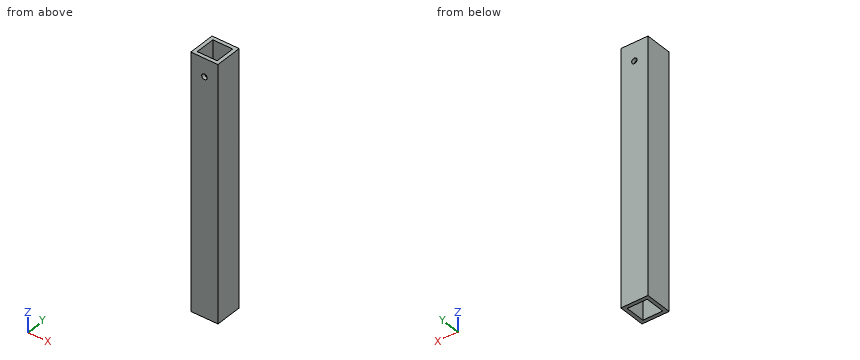
Autodesk Inventor part; units mm, degrees
ref_plane "YZ Plane" through (0, 0, 0) normal (1, 0, 0) x (0, 1, 0)
ref_plane "XZ Plane" through (0, 0, 0) normal (0, 1, 0) x (-1, 0, 0)
ref_plane "XY Plane" through (0, 0, 0) normal (0, 0, 1) x (1, 0, 0)
sketch "Sketch1" plane through (0, 0, 0) normal (0, 0, 1) x (1, 0, 0)
  line L0 (0, 0) -> (15, 0)
  line L1 (15, 0) -> (15, 15)
  line L2 (15, 15) -> (0, 15)
  line L3 (0, 15) -> (0, 0)
  dimension "d0" = 15
  dimension "d1" = 15
extrude "Extrusion1" add sketch "Sketch1" against normal blind 140
shell "Shell1" thickness 2 removed faces 2 at (10, 5, 0) at (10, 5, -140)
sketch "Sketch2" plane through (0, 15, 0) normal (0, 1, 0) x (1, 0, 0)
  line L0 (2, 0) -> (13, 0)
  line L1 (7.5, 0) -> (7.5, 10)
  circle A0 centre (7.5, 10) radius 1.5
  point P0 (0, 0)
  dimension "d5" = 10
  dimension "d6" = 3
extrude "Extrusion2" cut sketch "Sketch2" against normal through all
properties part number "Alumunium Square Tube 14cm"
Could you check a few things on this model? Use its own coordinates, in mm. Give positions to 0.01 mm unless a question says otherwise; leave off trailing zeros. Write each loop counter-clockwise with the first axis right and the second up, starting at its lowest first coordinate (ties: lowest second). Pieces come first, ordered by that corner, then holes. Notation, with made-up numbers: (24, -30) -> (40, -30) arc R31 cw to (40, -2) -> close; hole circle Ø6 at (64, -38.5). An arc over 180 degrees is marked (long way). Answer as a JSON object with one key per item and string values.
Q1. Suppose I cut it at C-C on z = -10. Write out the boundary of the cut face in (x, y).
Taken from the geometry:
{"outline": "(0, 0) -> (6, 0) -> (6, 2) -> (2, 2) -> (2, 13) -> (6, 13) -> (6, 15) -> (0, 15) -> close; (9, 0) -> (15, 0) -> (15, 15) -> (9, 15) -> (9, 13) -> (13, 13) -> (13, 2) -> (9, 2) -> close"}
Q2. Suppose I cut it at D-D on z = -130. Write out the boundary of the cut face in (x, y).
Taken from the geometry:
{"outline": "(0, 0) -> (15, 0) -> (15, 15) -> (0, 15) -> close; hole (2, 2) -> (13, 2) -> (13, 13) -> (2, 13) -> close"}
Q3. Please list where these lines run through material, in increasing order: L1, parallel to Y at x = 5, z = -30; L2, parallel to Z at x = 7.5, y = 1.35.
Taken from the geometry:
{"L1": "y = 0 to 2, 13 to 15", "L2": "z = -140 to -11.5, -8.5 to 0"}
Q4. Suppose I cut it at A-A on y = 11.75. Write out the boundary of the cut face in (x, z), then the cut area to 3 significant figures.
Taken from the geometry:
{"outline": "(0, -140) -> (2, -140) -> (2, 0) -> (0, 0) -> close; (13, -140) -> (15, -140) -> (15, 0) -> (13, 0) -> close", "area": "560 mm²"}
